Geometry check sheet. Reference: the model listing, model coordinates, mm. Face numbers are marked on the shaded views. Coordinates: 2 decimals unless noted, no trailing zeros. Loops run counter-clockwise (first coordinate to the right, second up) from the corner with the lowest first, then second, coordinate; pieces in that order, holes last. Notation, with made-up numbers: (87.5, -9.75) - (107.5, -9.75) arc R24 ccw to (107.5, 17.25) - close; hole circle Ø8 at (43, 58.5). An arc over 180 degrees is marked (long way). One line per item, written item: value.
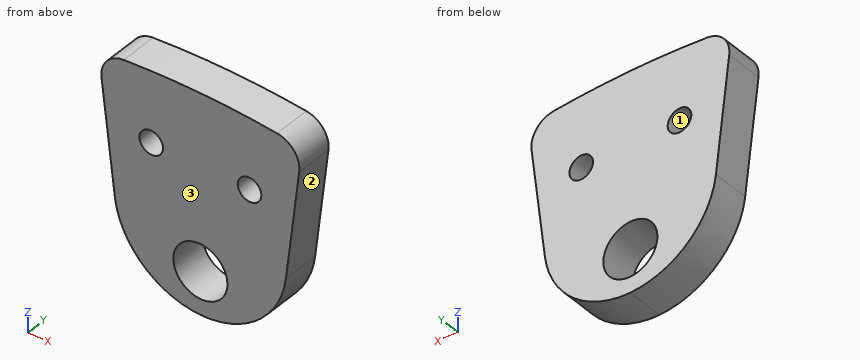
from build123d import *

# Parameters (mm, degrees)
SKETCH1_R            = 5.5
BOSS_EXTRUDE1_DEPTH  = 7.5
FILLET1_START        = -1
FILLET1_DEPTH        = 9
M4_CLEARANCE_HOLE1_D = 4.8
FILLET2_R            = 5


with BuildPart() as part:
    # Sketch1 → Boss-Extrude1 (new body)
    with BuildSketch(Plane(origin=(0, 0, 0), x_dir=(1, 0, 0), z_dir=(0, 1, 0))):
        with BuildLine():
            Line((-17.306036515, 15.320071712), (-20.703818553, -13.05219824))
            ThreePointArc((-20.703818553, -13.05219824), (0, -14.2875), (20.703818553, -13.05219824))
            Line((20.703818553, -13.05219824), (17.306036515, 15.320071712))
            Line((17.306036515, 15.320071712), (15.436394314, 30.932018749))
            ThreePointArc((15.436394314, 30.932018749), (0, 30.011), (-15.436394314, 30.932018749))
            Line((-15.436394314, 30.932018749), (-17.306036515, 15.320071712))
        make_face()
        with Locations(Location((0, 21.336, 0), (0, 0, 270))):
            Circle(SKETCH1_R, mode=Mode.SUBTRACT)
    extrude(amount=BOSS_EXTRUDE1_DEPTH)

    # Fillet1: read off the stored shape, not the designer's step
    # Fillet1 outline → Fillet1 (cut)
    with BuildSketch(Plane(origin=(0, 0, 0), x_dir=(1, 0, 0), z_dir=(0, 1, 0)).offset(FILLET1_START)):
        with BuildLine():
            Line((-15.436394314, 30.932018749), (-17.395311398, 14.574605686))
            add(Edge.make_bspline(
                [(-17.395311398, 14.574605686), (-16.419132346, 22.72592771), (-10.364461962, 30.010999958), (-7.1e-08, 30.011)],
                knots=[0, 0, 0, 0, 0.499999999, 0.499999999, 0.499999999, 0.499999999], degree=3, weights=[1, 0.706302503, 0.559453755, 0.559453754]))
            ThreePointArc((-7.1e-08, 30.011), (-7.731923227, 30.24145925), (-15.436394314, 30.932018749))
        make_face()
        with BuildLine():
            ThreePointArc((15.436394314, 30.932018749), (7.731923156, 30.241459246), (-7.1e-08, 30.011))
            add(Edge.make_bspline(
                [(-7.1e-08, 30.011), (10.364461892, 30.011000042), (16.41913234, 22.725927763), (17.395311398, 14.574605686)],
                knots=[0.499999999, 0.499999999, 0.499999999, 0.499999999, 1, 1, 1, 1], degree=3, weights=[0.559453754, 0.559453753, 0.706302502, 1]))
            Line((17.395311398, 14.574605686), (15.436394314, 30.932018749))
        make_face()
    extrude(amount=FILLET1_DEPTH, mode=Mode.SUBTRACT)

    # M4 Clearance Hole1 (through all)
    with Locations(Plane(origin=(0, 7.5, 0), x_dir=(1, 0, 0), z_dir=(0, 1, 0))):
        with Locations((-9.993476963, 0.312731325), (9.993476963, 0.312731325)):
            Hole(M4_CLEARANCE_HOLE1_D / 2)

    # Fillet2
    fillet2_edges = [part.edges().sort_by_distance(p)[0] for p in [
        (20.703818553, 3.75, 13.05219824),
        (-20.703818553, 3.75, 13.05219824),
    ]]
    fillet(fillet2_edges, radius=FILLET2_R)


solid = part.part
(1) Cross-section at B-B on z = -4. Record the cut outline in (x, y).
Reply:
outline: (-18.66, 0) - (18.66, 0) - (18.66, 7.5) - (-18.66, 7.5) - close
(2) Go/stop test with flat-tipped pins: pin 1 Ø1.5 at (x, y) = (-3.5, 5) entering from -Z; pin 2 Ø1.5 at (y, z) = (3.5, 0) entering from +X; pin 3 Ø3 at (x, z) = (9.99, -0.31) entering from +Y. Record where each tip stops, or that it passes through.
Reply:
pin 1: z = -29.79
pin 2: x = 19.23
pin 3: through
(3) Cross-section at A-A on y = 3.25. State how many separate pieces and enclosed holes the cut face has, and give its area (3 significant figures).
Reply:
separate pieces: 1
enclosed holes: 3
area: 1,350 mm2
(4) Material ranges on probe 1 along X at (y, z) = (5.5, -14.5); probe 2 along X at (y, z) = (4.25, -17); probe 3 along X at (y, z) = (7.25, -22.5), recorded low to high. Write a range as from..to.
Reply:
probe 1: -17.4..17.4
probe 2: -16.93..-3.38, 3.38..16.93
probe 3: -14.38..-5.38, 5.38..14.38
(5) Release check for a two-part mould opening along Z. For the marked faces 1, 2 and 3 record: pulls with the +Z half, pulls with the -Z half, needs draft (parallel to the pull), parting line crosses it, or undercut.
Reply:
face 1: undercut
face 2: pulls with the -Z half
face 3: needs draft
